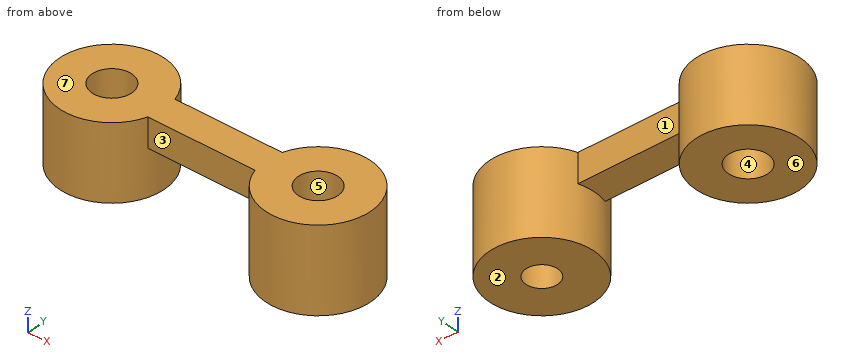
Autodesk Fusion 360 part; units mm, degrees
sketch "Sketch1" plane through (0, 0, 0) normal (0, 0, 1) x (1, 0, 0)
  circle A0 centre (0, 0) radius 4.5
  line L0 (0, 0) -> (17.87, 0) construction
  circle A1 centre (17.87, 0) radius 4.5
  line L1 (13.5773, 1.35) -> (4.2927, 1.35)
  line L2 (13.5773, -1.35) -> (4.2927, -1.35)
  dimension "d1" = 9
  dimension "d2" = 17.87
  dimension "d3" = 9
  dimension "d4" = 2.7
  dimension "d5" = 1.35
extrude "Extrude1" add sketch "Sketch1" along normal blind 6.4 contours A0 makes body 1
sketch "Sketch2" plane through (0, 0, 6.4) normal (0, 0, 1) x (-1, 0, 0)
  circle A0 centre (0, 0) radius 4.5
  line L0 (0, 0) -> (-17.87, 0) construction
  circle A1 centre (-17.87, 0) radius 4.5
  dimension "d8" = 17.87
  dimension "d9" = 9
extrude "Extrude2" add sketch "Sketch2" against normal blind 7.2 separate body contours A1 makes body 2
sketch "Sketch3" plane through (0, 0, 6.4) normal (0, 0, 1) x (-1, 0, 0)
  circle A0 centre (0, 0) radius 4.5
  circle A1 centre (0, 0) radius 4.5
  line L0 (0, 0) -> (-17.87, 0) construction
  circle A2 centre (-17.87, 0) radius 4.5
  line L1 (-4.2925, -1.3507) -> (-13.5775, -1.3507)
  line L2 (-13.5775, 1.3507) -> (-4.2925, 1.3507)
  dimension "d12" = 17.87
  dimension "d13" = 9
  dimension "d14" = 9.285
  dimension "d15" = 9.285
extrude "Extrude3" add sketch "Sketch3" against normal blind 2.49 contours A0 A1 A2 L1 L2 bodies 1 2
sketch "Sketch4" plane through (0, 0, 0) normal (0, 1, 0) x (1, 0, 0)
hole "Hole1" at (0, 0, 6.4) direction (0, 0, -1) diameter 3.4 depth 7 tip angle 118 bodies 1
hole "Hole2" at (17.87, 0, 6.4) direction (0, 0, -1) diameter 3.4 depth 7 tip angle 118 bodies 1
Model file for the job. Use its own axes, mm. Face numbers are marked on the shaded views. A direction names the side the tool comes from. Coordinates: 2 decimals unless noted, no trailing zeros. Loops run counter-clockwise (first coordinate to the right, second up) from the corner with the lowest first, then second, coordinate; pieces in that order, holes last. Notation, with made-up numbers: (7.25, -3.75) -> (37.25, -3.75) arc R32 ccw to (37.25, 26.25) -> close; hole circle Ø11 at (59.25, 8). An arc over 180 degrees is marked (long way). Answer as a JSON object with one key per item and string values.
Q1. Cut at D-D (y = 0). List the corners of the cut face in (x, z).
Report:
{"outline": "(-4.5, 0) -> (-1.7, 0) -> (-1.7, 6.4) -> (-4.5, 6.4) -> close; (1.7, 0) -> (4.5, 0) -> (4.5, 3.91) -> (13.37, 3.91) -> (13.37, -0.8) -> (16.5, -0.8) -> (16.17, -0.6) -> (16.17, 6.4) -> (1.7, 6.4) -> close; (19.24, -0.8) -> (22.37, -0.8) -> (22.37, 6.4) -> (19.57, 6.4) -> (19.57, -0.6) -> close"}
Q2. Pull direction Y, two halves, no side cores. Call the marked faces 1, 2, 3 and 4: released by +Y, released by -Y, zero draft, split by the parting line, or undercut.
Report:
{"face 1": "released by +Y", "face 2": "zero draft", "face 3": "released by -Y", "face 4": "undercut"}
Q3. 3-axis set-ups, long thin cutter, end or side, ignore diameter. For the marked faces 5, 6 and 7: which of +Z, -Z, +X, -X, +Y, -Y reach the whole face in a straight line?
Report:
{"face 5": "+Z", "face 6": "-Z, -X, +Y, -Y", "face 7": "+Z, +X, -X, +Y, -Y"}
Q4. Cut at B-B (x = 17.87). List the corners of the cut face in (y, z), and give its area (3 significant figures).
Report:
{"outline": "(-4.5, -0.8) -> (-1.37, -0.8) -> (-1.7, -0.6) -> (-1.7, 6.4) -> (-4.5, 6.4) -> close; (1.37, -0.8) -> (4.5, -0.8) -> (4.5, 6.4) -> (1.7, 6.4) -> (1.7, -0.6) -> close", "area": "40.4 mm2"}
Q5. Flat gauge pins, fed straight in: P1, Ø2, axis at y = 3.5, z = 3.5, coming from the +X side; P2, Ø4.5, axis at x = 0.5, y = 0.5, coming from the -Z side; P3, Ø1, axis at x = 4, z = 1, coming from the +Y side; P4, Ø2, axis at x = 0, y = 0, coming from the -Z side. Where does each tip first touch, or does it go through?
Report:
{"P1": "stops at x = 21.61", "P2": "stops at z = 0", "P3": "stops at y = 2.83", "P4": "passes through"}
Q6. Cut at A-A (z = 0.75). List the corners of the cut face in (x, y).
Report:
{"outline": "circle Ø9 at (0, 0); circle Ø9 at (17.87, 0); hole circle Ø3.4 at (0, 0); hole circle Ø3.4 at (17.87, 0)"}
Q7. Cut at C-C (y = -3.5). List the corners of the cut face in (x, z).
Report:
{"outline": "(-2.83, 0) -> (2.83, 0) -> (2.83, 6.4) -> (-2.83, 6.4) -> close; (15.04, -0.8) -> (20.7, -0.8) -> (20.7, 6.4) -> (15.04, 6.4) -> close"}
Q8. Probe probe 1 along X at (y, z) = (0, 3); probe 2 along X at (y, z) = (0, 4); probe 3 along Y at (x, z) = (17.87, 2). List the from-to ranges inside material, lowest first.
Report:
{"probe 1": "x = -4.5 to -1.7, 1.7 to 4.5, 13.37 to 16.17, 19.57 to 22.37", "probe 2": "x = -4.5 to -1.7, 1.7 to 16.17, 19.57 to 22.37", "probe 3": "y = -4.5 to -1.7, 1.7 to 4.5"}
